For this review, use the dimensioned drawing (mm, ordinates from the lowest corner) and the shaded views. A direction names the side the tool comes from. Coordinates: 2 decimals unless noted, no trailing zeros. Write each loop counter-clockwise with the first axis right and the second up, starting at its lowest first coordinate (ties: lowest second). Pieces come first, ordered by that corner, then holes. Notation, with made-up numbers: M 10.5,-3 L 40.5,-3 A22 ccw 40.5,34 Z; hole C 73,-26.75 d1. An arc over 180 degrees is marked long. One line per question, with ' | ' between items.
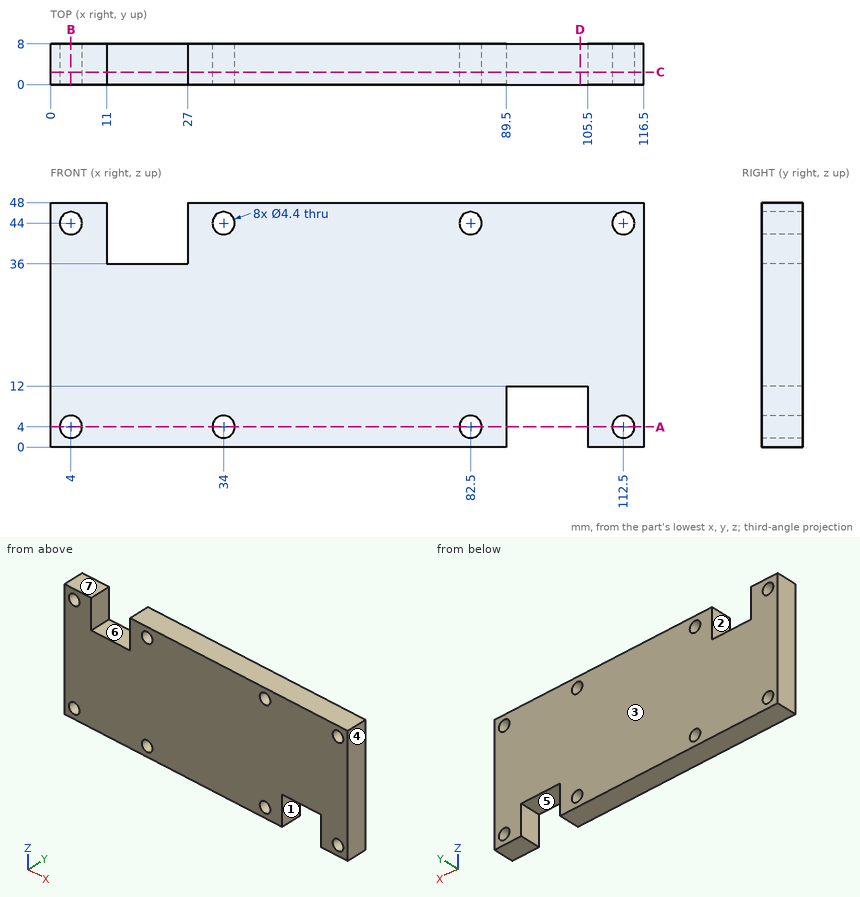
1) Insertion check: pin 1 Ø4 at (x, z) = (112.5, 4) entering from +Y; pin 2 Ø2.5 at (x, y) = (15.5, 2.5) entering from +Z; pin 3 Ø3 at (x, y) = (101.5, 6.5) entering from -Z. Each pin has a flat end and moves straight along its axis. Give the tip position at first contact, or say it passes through.
Responses:
pin 1: through | pin 2: z = 36 | pin 3: z = 12
2) The part is to be moulded in two halves that separate along X. For the marked faces 1, 2, 3 and 4, say which applies: +X half, -X half, draft (parallel to the pull), parting line (faces both ways), or undercut.
Responses:
face 1: undercut | face 2: undercut | face 3: draft | face 4: +X half
3) We need section D-D on x = 104. State the section outline as (y, z) points.
Responses:
outline: M 0,12 L 8,12 L 8,48 L 0,48 Z
4) We need section C-C on y = 2.5. State how many separate pieces and enclosed holes the cut face has, then the cut area to 3 significant figures.
Responses:
separate pieces: 1 | enclosed holes: 8 | area: 5,090 mm^2
5) We need section B-B on x = 4. State the section outline as (y, z) points, then the cut area to 3 significant figures.
Responses:
outline: M 0,0 L 8,0 L 8,1.8 L 0,1.8 Z; M 0,6.2 L 8,6.2 L 8,41.8 L 0,41.8 Z; M 0,46.2 L 8,46.2 L 8,48 L 0,48 Z | area: 314 mm^2
6) To check wall thickness, follow line 1 along Z through (x, y) = (82.5, 3.75); line 2 along X through (y, z) = (3.75, 41); line 3 along X through (y, z) = (4.75, 3). State the ranges of each line that lie inside material, in increasing order. Write a range as [from, to].
Responses:
line 1: [0, 1.8], [6.2, 41.8], [46.2, 48] | line 2: [0, 11], [27, 116.5] | line 3: [0, 2.04], [5.96, 32.04], [35.96, 80.54], [84.46, 89.5], [105.5, 110.54], [114.46, 116.5]
7) Machinability: for the marked faces 5, 6 and 7, which of the approach directions +Z, -Z, +X, -X, +Y, -Y give a long, thin tool a straight path to every point of the face, cutting with its end or side? Answer none if there is none.
Responses:
face 5: -Z, +Y, -Y | face 6: +Z, +Y, -Y | face 7: +Z, +X, -X, +Y, -Y
8) We need section A-A on z = 4. State the section outline as (x, y) points.
Responses:
outline: M 0,0 L 1.8,0 L 1.8,8 L 0,8 Z; M 6.2,0 L 31.8,0 L 31.8,8 L 6.2,8 Z; M 36.2,0 L 80.3,0 L 80.3,8 L 36.2,8 Z; M 84.7,0 L 89.5,0 L 89.5,8 L 84.7,8 Z; M 105.5,0 L 110.3,0 L 110.3,8 L 105.5,8 Z; M 114.7,0 L 116.5,0 L 116.5,8 L 114.7,8 Z
